from build123d import *

# Parameters (mm, degrees)
SKETCH_R  = 6.5
PAD_DEPTH = 8


with BuildPart() as part:
    # Sketch → Pad (new body)
    with BuildSketch(Plane.XY):
        with BuildLine():
            ThreePointArc((-28.769231, -18.119916), (-16.430503, -29.7664), (0, -34))
            Line((0, -34), (33, -34))
            ThreePointArc((38, -39), (36.535534, -35.464466), (33, -34))
            Line((38, -39), (38, -76))
            ThreePointArc((33, -81), (36.535534, -79.535534), (38, -76))
            Line((-33, -81), (33, -81))
            ThreePointArc((-38, -76), (-36.535534, -79.535534), (-33, -81))
            Line((-38, -20.78461), (-38, -76))
            ThreePointArc((-28.769231, -18.119916), (-34.38675, -15.980765), (-38, -20.78461))
        make_face()
        with Locations((-25, -50)):
            Circle(SKETCH_R, mode=Mode.SUBTRACT)
        with Locations((25, -67)):
            Circle(SKETCH_R, mode=Mode.SUBTRACT)
    extrude(amount=PAD_DEPTH)


solid = part.part
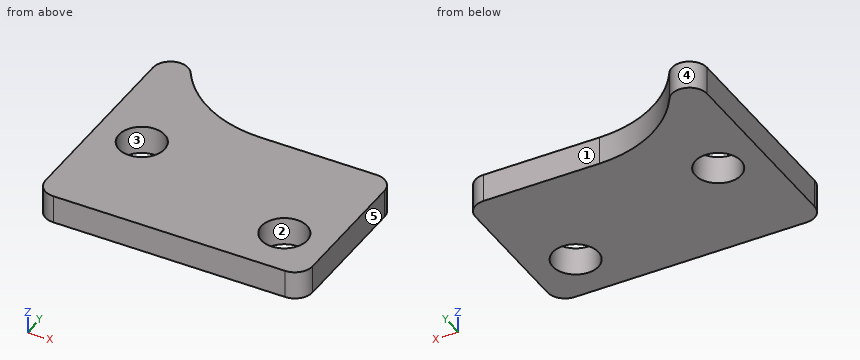
Design review of the part built by this model. Coordinates are the model's own, in mm. Face numbers are marked on the shaded views. A direction names the side the tool comes from. Round coordinates to 2 decimals unless told otherwise and drop trailing zeros. Write each loop counter-clockwise with the first axis right and the second up, starting at its lowest first coordinate (ties: lowest second). Pieces come first, ordered by that corner, then holes. Notation, with made-up numbers: (-14.75, 13.25) - (16.25, 13.25) arc R32 cw to (16.25, 51.25) - close; hole circle Ø8 at (84, 19.25). An arc over 180 degrees is marked (long way). Use a Markdown table: item, result. Add a question column.
1. We need section A-A (y = -52.5). State the section outline as (x, z) points, then the cut area to 3 significant figures.
2. Wall thickness on probe 1 along Y at (x, z) = (25, 4.5); probe 2 along Y at (x, z) = (23.5, 0.5); probe 3 along X at (y, z) = (-66.5, 1.5): over which ranges is each line inside the solid? List them lowest first.
3. We need section B-B (z = 2.5). State the section outline as (x, y) points, then the cut area to 3 significant figures.
4. Clearance check with flat-ended pins moving along their axes: pin 1 (21 mm diameter, centred on x = -25, y = -50, fed in from +Z); pin 2 (3 mm diameter, centred on y = -35, z = 6.5, fed in from +X); pin 3 (1 mm diameter, centred on x = 5, z = 2.5, fed in from +Y). State where each tip first meets the part, or that it passes through.
5. We need section C-C (x = 25). State the section outline as (y, z) points.
6. Mouldability with a two-part tool opening along Y and no side actions: class the marked faces 3, 4 and 5 as +Y half, -Y half, draft (parallel to the pull), parting line (faces both ways), or undercut.
7. For the marked faces 1 and 2, list the 3-axis set-ups (+Z, -Z, +X, -X, +Y, -Y) from which the entire face can be reached by the end or side of a thin tool; tool diameter is ignored.
8. We need section D-D (x = -17.5). State the section outline as (y, z) points.
Output:
| question | item | result |
|---|---|---|
| 1 | outline | (-38, 0) - (-31, 0) - (-31, 8) - (-38, 8) - close; (-19, 0) - (38, 0) - (38, 8) - (-19, 8) - close |
| 1 | area | 512 mm2 |
| 2 | probe 1 | y = -81 to -73.5, -60.5 to -34 |
| 2 | probe 2 | y = -81 to -73.32, -60.68 to -34 |
| 2 | probe 3 | x = -38 to 18.52, 31.48 to 38 |
| 3 | outline | (-38, -76) arc R5 ccw to (-33, -81) - (33, -81) arc R5 ccw to (38, -76) - (38, -39) arc R5 ccw to (33, -34) - (0, -34) arc R34 cw to (-28.77, -18.12) arc R5 ccw to (-38, -20.78) - close; hole circle Ø13 at (-25, -50); hole circle Ø13 at (25, -67) |
| 3 | area | 3,580 mm2 |
| 4 | pin 1 | stops at z = 8 |
| 4 | pin 2 | stops at x = 37.33 |
| 4 | pin 3 | stops at y = -34 |
| 5 | outline | (-81, 0) - (-73.5, 0) - (-73.5, 8) - (-81, 8) - close; (-60.5, 0) - (-34, 0) - (-34, 8) - (-60.5, 8) - close |
| 6 | face 3 | undercut |
| 6 | face 4 | +Y half |
| 6 | face 5 | draft |
| 7 | face 1 | +Z, -Z, +X, +Y |
| 7 | face 2 | +Z, -Z |
| 8 | outline | (-81, 0) - (-29.15, 0) - (-29.15, 8) - (-81, 8) - close |
